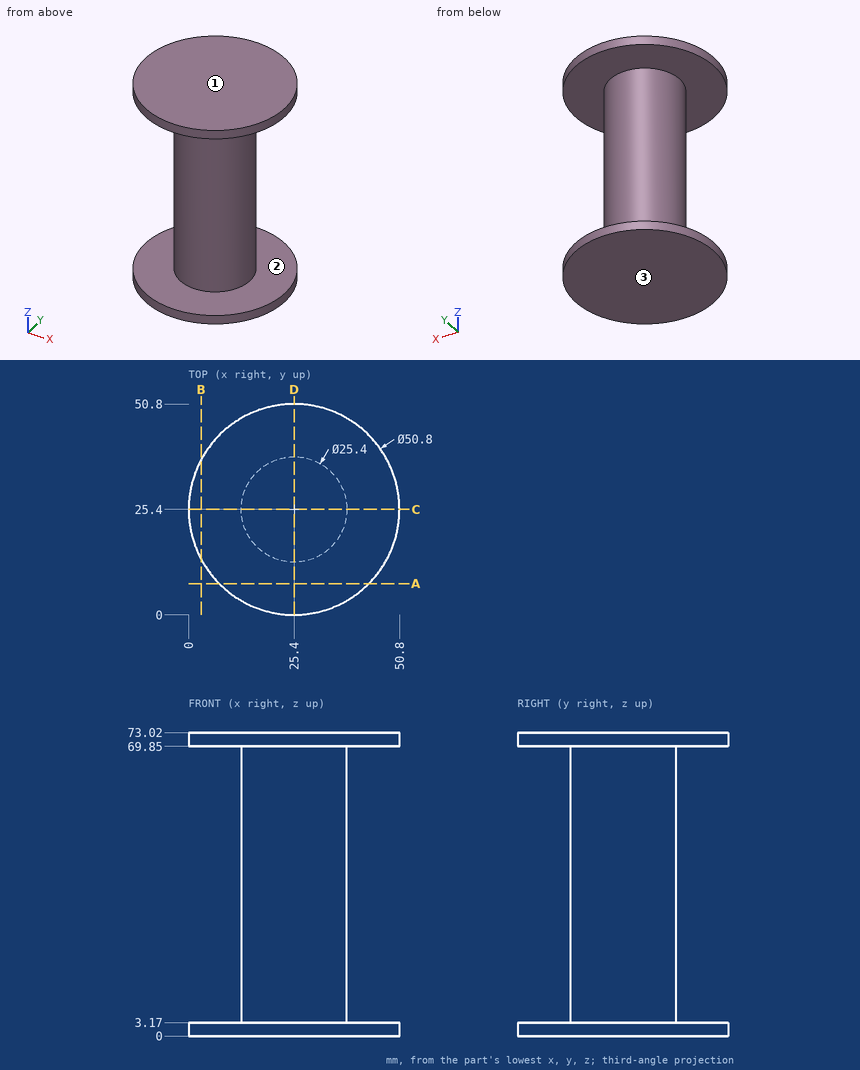
Could you check a few things on this drawing? It's one solid part, dimensions in mm from its lowest x, y, z. Round coordinates to 2 decimals unless told otherwise and drop trailing zeros. Order: outer loops, then holes, each group sorted by start corner. A loop starts at its lowest first (then second) coordinate and runs counter-clockwise, first axis right, second up. Notation, with made-up numbers: M 50,54.5 L 100,54.5 A20 cw 100,77.5 Z; hole C -16,39 d10. An arc over 180 degrees is marked long. Use a Markdown table: item, result.
1) Imagine slicing it at C-C (y = 25.4). List the corners of the cut face in (x, z) for me, then the cut area to 3 significant figures.
Geometry says:
| item | result |
|---|---|
| outline | M 0,0 L 50.8,0 L 50.8,3.17 L 38.1,3.17 L 38.1,69.85 L 50.8,69.85 L 50.8,73.02 L 0,73.02 L 0,69.85 L 12.7,69.85 L 12.7,3.17 L 0,3.17 Z |
| area | 2,020 mm² |
2) I'm going to push flat-ended pins straight in: P1, Ø5, axis at y = 39.5, z = 49.5, coming from the -X side; P2, Ø4, axis at y = 10.5, z = 57, coming from the -X side; P3, Ø12, axis at x = 23, z = 41.5, coming from the +Y side; P4, Ø10, axis at x = 18, z = 16.5, coming from the -Y side. Where does each tip first touch, or does it pass through?
Geometry says:
| item | result |
|---|---|
| P1 | stops at x = 20.23 |
| P2 | passes through |
| P3 | stops at y = 38.1 |
| P4 | stops at y = 12.93 |
3) If I drill on line 1 along Z through (x, y) = (48, 34); line 2 along Y through (x, z) = (35, 67); line 3 along Y through (x, z) = (21, 37), over which ranges is the centre line in solid material (lowest first)?
Geometry says:
| item | result |
|---|---|
| line 1 | z = 0 to 3.17, 69.85 to 73.02 |
| line 2 | y = 17.09 to 33.71 |
| line 3 | y = 13.49 to 37.31 |
4) Imagine slicing it at A-A (y = 7.5). List the corners of the cut face in (x, z) for me.
Geometry says:
| item | result |
|---|---|
| outline | M 7.38,0 L 43.42,0 L 43.42,3.17 L 7.38,3.17 Z; M 7.38,69.85 L 43.42,69.85 L 43.42,73.02 L 7.38,73.02 Z |
5) Imagine slicing it at B-B (x = 3). List the corners of the cut face in (y, z) for me.
Geometry says:
| item | result |
|---|---|
| outline | M 13.43,0 L 37.37,0 L 37.37,3.17 L 13.43,3.17 Z; M 13.43,69.85 L 37.37,69.85 L 37.37,73.02 L 13.43,73.02 Z |
6) If we mould it in two halves opening along Z, with no side actions, what happens to the marked faces 1, 2 and 3? For each: +Z half, -Z half, draft (parallel to the pull), parting line (faces both ways), or undercut.
Geometry says:
| item | result |
|---|---|
| face 1 | +Z half |
| face 2 | undercut |
| face 3 | -Z half |
